For this review, take the finished solid that the model builds, in its own axes (mm). A direction names the side the tool comes from. Coordinates: 2 decimals unless noted, no trailing zeros. Loops run counter-clockwise (first coordinate to the right, second up) from the corner with the lowest first, then second, coordinate; pieces in that order, holes last. Notation, with made-up numbers: M 24,-26.5 L 50,-26.5 A18 cw 50,8.5 Z; hole C -3,33 d1. An arc over 180 degrees is marked long. Write each question's results on one line, items separated by ' | '. Start each with the question number.
```python
from build123d import *

# Parameters (mm, degrees)
BOSS_EXTRUDE1_DEPTH = 7
SKETCH3_R           = 1.6
CUT_EXTRUDE1_DEPTH  = 7
FILLET1_R           = 5
FILLET2_R           = 2


with BuildPart() as part:
    # Sketch2 → Boss-Extrude1 (new body)
    with BuildSketch(Plane.XY):
        Polygon((-25, 1.5), (-25, -1.5), (25, -1.5), (25, 1.5), (15, 1.5), (12, 1.5), (-12, 1.5), (-15, 1.5), align=None)
        Polygon((-15, 16.783591394), (-15, 1.5), (-12, 1.5), (-12, 13.783591394), (12, 13.783591394), (12, 1.5), (15, 1.5), (15, 16.783591394), align=None)
    extrude(amount=BOSS_EXTRUDE1_DEPTH)

    # Sketch3 → Cut-Extrude1 (cut)
    with BuildSketch(Plane(origin=(0, 1.5, 0), x_dir=(1, 0, 0), z_dir=(0, 1, 0))):
        with Locations(Location((-20, -3.5, 0), (0, 0, 270))):
            Circle(SKETCH3_R)
        with Locations(Location((20, -3.5, 0), (0, 0, 270))):
            Circle(SKETCH3_R)
    extrude(amount=-CUT_EXTRUDE1_DEPTH, mode=Mode.SUBTRACT)

    # Fillet1
    fillet1_edges = [part.edges().sort_by_distance(p)[0] for p in [
        (-15, 16.783591394, 3.5),
        (15, 16.783591394, 3.5),
        (12, 13.783591394, 3.5),
        (-12, 13.783591394, 3.5),
    ]]
    fillet(fillet1_edges, radius=FILLET1_R)

    # Fillet2
    fillet2_edges = [part.edges().sort_by_distance(p)[0] for p in [
        (-25, 0, 0),
        (25, 0, 0),
        (-15, 1.5, 3.5),
        (15, 1.5, 3.5),
        (25, 0, 7),
        (-25, 0, 7),
    ]]
    fillet(fillet2_edges, radius=FILLET2_R)


solid = part.part
```
Q1. For faces 1 (the face through (15, 8, 3)), 2 (the face through (-15, 8, 3)), 3 (the face through (-10.574, 12.28, 3.549)), list the 3-axis set-ups (+Z, -Z, +X, -X, +Y, -Y) from which the entire face can be reached by the end or side of a thin tool; tool diameter is ignored.
Q2. Take a section at B-B, the plane y = 5. Give the boundary of the cut face in (x, z).
Q3. Take a section at D-D, the plane z = 6.25. Give the boundary of the cut face in (x, y), then the cut area to 3 significant figures.
Q4. The part is to be moulded in two halves that separate along Z. For faces 4 (the face through (0, 0, 7)), 5 (the face through (-22, 1.5, 3)), 6 (the face through (-24.4, -0.02, 0.57)), 7 (the face through (-18.414, 0.021, 3.292)), say which applies: pulls with the +Z half, pulls with the -Z half, needs draft (parallel to the pull), parting line crosses it, or undercut.
Q5. Take a section at C-C, the plane x = -6. Give the boundary of the cut face in (y, z).
Q6. To check wall thickness, follow line 1 along X through (y, z) = (-0.05, 3.5); line 2 along Y through (x, z) = (-2, 1); line 3 along X through (y, z) = (9, 1.5). State the ranges of each line that lie inside material, in increasing order.
Q7. Insertion check: P1, Ø2.5, axis at x = -20, z = 3.5, coming from the +Y side; P2, Ø2, axis at y = 9.5, z = 4, coming from the -X side. Each pin has a flat end and moves straight along its axis. Give the tip position at first contact, or say it passes through.
Q8. Take a section at A-A, the plane z = 3.5. Give the boundary of the cut face in (x, y), then the cut area to 3 significant figures.
Results:
1) face 1: +Z, -Z, +X, +Y | face 2: +Z, -Z, -X, +Y | face 3: +Z, -Z
2) outline: M -15,0 L -12,0 L -12,7 L -15,7 Z; M 12,0 L 15,0 L 15,7 L 12,7 Z
3) outline: M -24.56,-1.5 L 24.56,-1.5 L 24.56,1.5 L 17,1.5 A2 cw 15,3.5 L 15,11.78 A5 ccw 10,16.78 L -10,16.78 A5 ccw -15,11.78 L -15,3.5 A2 cw -17,1.5 L -24.56,1.5 Z; hole M -12,1.5 L 12,1.5 L 12,8.78 A5 ccw 7,13.78 L -7,13.78 A5 ccw -12,8.78 Z | area: 313 mm^2
4) face 4: pulls with the +Z half | face 5: needs draft | face 6: pulls with the -Z half | face 7: undercut
5) outline: M -1.5,0 L 1.5,0 L 1.5,7 L -1.5,7 Z; M 13.78,0 L 16.78,0 L 16.78,7 L 13.78,7 Z
6) line 1: -25 to -21.6, -18.4 to 18.4, 21.6 to 25 | line 2: -1.5 to 1.5, 13.78 to 16.78 | line 3: -15 to -12, 12 to 15
7) P1: through | P2: x = -15
8) outline: M -25,-1.5 L -21.6,-1.5 L -21.6,1.5 L -25,1.5 Z; M -18.4,-1.5 L 18.4,-1.5 L 18.4,1.5 L 17,1.5 A2 cw 15,3.5 L 15,11.78 A5 ccw 10,16.78 L -10,16.78 A5 ccw -15,11.78 L -15,3.5 A2 cw -17,1.5 L -18.4,1.5 Z; M 21.6,-1.5 L 25,-1.5 L 25,1.5 L 21.6,1.5 Z; hole M -12,1.5 L 12,1.5 L 12,8.78 A5 ccw 7,13.78 L -7,13.78 A5 ccw -12,8.78 Z | area: 296 mm^2
